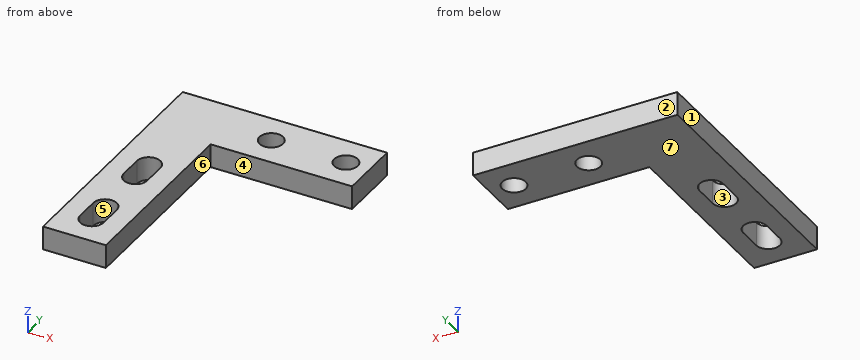
Autodesk Inventor part; units mm, degrees
ref_plane "YZ Plane" through (0, 0, 0) normal (1, 0, 0) x (0, 1, 0)
ref_plane "XZ Plane" through (0, 0, 0) normal (0, 1, 0) x (-1, 0, 0)
ref_plane "XY Plane" through (0, 0, 0) normal (0, 0, 1) x (1, 0, 0)
sketch "Sketch1" plane through (0, 0, 0) normal (0, 0, 1) x (1, 0, 0)
  line L0 (-4, -24) -> (-4, 8)
  line L1 (-4, 8) -> (22, 8)
  line L2 (22, 8) -> (22, 0)
  line L3 (22, 0) -> (4, 0)
  line L4 (4, 0) -> (4, -24)
  line L5 (4, -24) -> (-4, -24)
  point P0 (0, 0)
  dimension "d0" = 0
  dimension "d1" = 8
  dimension "d2" = 8
  dimension "d3" = 4
  dimension "d5" = 26
  dimension "d6" = 32
extrude "Extrusion1" add sketch "Sketch1" along normal blind 3
sketch "Sketch2" plane through (0, 0, 3) normal (0, 0, 1) x (1, 0, 0)
  circle A0 centre (0, 4) radius 1.5
  circle A1 centre (19, 4) radius 1.5
  circle A2 centre (0, -6) radius 1.5
  circle A3 centre (9.5, 4) radius 1.5
  line L0 (-4, 8) -> (-4, -24)
  point P0 (0, 0)
  dimension "d9" = 3
  dimension "d10" = 3
  dimension "d11" = 3
  dimension "d12" = 10
  dimension "d15" = 4
  dimension "d24" = 9.5
  dimension "d25" = 13.5
hole "Hole1" at (9.5, 4, 3) at (19, 4, 3) direction (0, 0, -1) diameter 3 end through all
sketch "Sketch3" plane through (0, 0, 3) normal (0, 0, 1) x (1, 0, 0)
  line L0 (0, -7) -> (0, -10) construction
  line L1 (-1.5, -7) -> (-1.5, -10)
  line L2 (1.5, -10) -> (1.5, -7)
  arc A0 (1.5, -7) -> (-1.5, -7) centre (0, -7) ccw
  arc A1 (-1.5, -10) -> (1.5, -10) centre (0, -10) ccw
  line L3 (0, -17) -> (0, -20) construction
  line L4 (-1.5, -17) -> (-1.5, -20)
  line L5 (1.5, -20) -> (1.5, -17)
  arc A2 (1.5, -17) -> (-1.5, -17) centre (0, -17) ccw
  arc A3 (-1.5, -20) -> (1.5, -20) centre (0, -20) ccw
  point P0 (0, 0)
  point P1 (0, -8.5)
  point P2 (0, -18.5)
  dimension "d26" = 3
  dimension "d27" = 3
  dimension "d29" = 10
  dimension "d32" = 7
extrude "Extrusion2" cut sketch "Sketch3" against normal through all
equation "\"d16\" = d11"
properties part number "Gripper_Endstop_Holder" material "Aluminum 6061"
Geometry: final body of the model. Coordinates: model frame, mm. Face numbers are marked on the shaded views. A direction names the side the tool comes from. Coordinates: 2 decimals unless noted, no trailing zeros. Loops run counter-clockwise (first coordinate to the right, second up) from the corner with the lowest first, then second, coordinate; pieces in that order, holes last. Notation, with made-up numbers: (-18.5, 21.5) - (-7.5, 21.5) arc R18 ccw to (-7.5, 56.5) - close; hole circle Ø1 at (52.5, -20.75). An arc over 180 degrees is marked (long way). Put each result on its own line as item: value. Start each with the question number.
Q1. Cut plane B-B, the plane y = 4. Return loops of the section in (x, z).
Q2. Line query: line 1 (X direction, y = 4, z = 0.8); line 2 (Y direction, x = 9.5, z = 1.05); line 3 (X direction, y = -9, z = 1.95). Output: solid intervals per line, ascending.
Q3. Cut plane C-C, the plane z = 0.55. Return loops of the section in (x, y), and give its area (3 significant figures).
Q4. Pull-direction query (Y, two-part tool) for the marked faces 1, 2, 3 and 4; classes: released by +Y, released by -Y, zero draft, split by the parting line, or undercut.
Q5. Set-up query: the marked faces 5, 6 and 7. Return all of +Z, -Z, +X, -X, +Y, -Y with unobstructed straight access to the full face (end or side cutting, diameter ignored); none if empty.
Q6. Cut plane A-A, the plane x = 9.5. Return loops of the section in (y, z), and give its area (3 significant figures).
Q7. Cut plane D-D, the plane y = -16.5. Return loops of the section in (x, z).
Q8. Pin query (flat end, axial travel): pin 1 Ø1.8 at (x, y) = (9.5, 4) entering from -Z; pin 2 Ø4 at (x, y) = (19, 4) entering from +Z. Return the tip coordinate at first contact, or that it passes through.
Filled sheet:
1. outline: (-4, 0) - (8, 0) - (8, 3) - (-4, 3) - close; (11, 0) - (17.5, 0) - (17.5, 3) - (11, 3) - close; (20.5, 0) - (22, 0) - (22, 3) - (20.5, 3) - close
2. line 1: -4 to 8, 11 to 17.5, 20.5 to 22
2. line 2: 0 to 2.5, 5.5 to 8
2. line 3: -4 to -1.5, 1.5 to 4
3. outline: (-4, -24) - (4, -24) - (4, 0) - (22, 0) - (22, 8) - (-4, 8) - close; hole (-1.5, -20) arc R1.5 ccw to (1.5, -20) - (1.5, -17) arc R1.5 ccw to (-1.5, -17) - close; hole (-1.5, -10) arc R1.5 ccw to (1.5, -10) - (1.5, -7) arc R1.5 ccw to (-1.5, -7) - close; hole circle Ø3 at (9.5, 4); hole circle Ø3 at (19, 4)
3. area: 354 mm²
4. face 1: zero draft
4. face 2: released by +Y
4. face 3: undercut
4. face 4: released by -Y
5. face 5: +Z, -Z
5. face 6: +Z, -Z, +X, -Y
5. face 7: -Z, +X, -X, +Y, -Y
6. outline: (0, 0) - (2.5, 0) - (2.5, 3) - (0, 3) - close; (5.5, 0) - (8, 0) - (8, 3) - (5.5, 3) - close
6. area: 15.0 mm²
7. outline: (-4, 0) - (-1.41, 0) - (-1.41, 3) - (-4, 3) - close; (1.41, 0) - (4, 0) - (4, 3) - (1.41, 3) - close
8. pin 1: through
8. pin 2: z = 3
